Can you work these out from the model? Positions are in its coordinate system, mm. A direction names the side the tool comes from. Give positions to 0.01 mm unless a question says otherwise; leave off trailing zeros. Use a Markdown table: item, result. Add a question column.
```python
from build123d import *

# Parameters (mm, degrees)
F0_W      = 2.5
F0_H      = 4.3
F1_DEPTH  = 0.01
F4_W      = 3
F4_H      = 2.4
F5_DEPTH  = 2
F0_W_2    = 0.25
F0_H_2    = 26.2
F6_DEPTH  = 0.01
F7_DEPTH  = 0.01
F7_FACE_W = 0.25
F7_FACE_H = 28.7
F6_FACE_W = 0.25
F6_FACE_H = 26.2
F10_R     = 0.2
F11_W     = 38
F11_H     = 33
F12_DEPTH = 12.5


with BuildPart() as f1:
    # F0 (on Front) → F1 (new body)
    with BuildSketch(Plane.XZ):
        with Locations((1.25, 2.15)):
            Rectangle(F0_W, F0_H)
        Polygon((2.5, 0), (0, 0), (0, -1), (1.02, -1), (1.27, -1), (2.9, -1), (2.9, 0), align=None)
    extrude(amount=F1_DEPTH)

    # F1_face (on face) → F2 (revolve)
    with BuildSketch(Plane(origin=(1.2924908425, -0.01, 1.586996337), x_dir=(1, 0, 0), z_dir=(0, -1, 0))):
        Polygon((-1.2924908425, 2.713003663), (-1.2924908425, -2.586996337), (1.6075091575, -2.586996337), (1.6075091575, -1.586996337), (1.2075091575, -1.586996337), (1.2075091575, 2.713003663), align=None)
    revolve(axis=Axis((0, 0, 1.65), (0, 0, 1)))

    # F4 (on offset) → F5 (cut)
    with BuildSketch(Plane.YZ.offset(2.5)):
        Rectangle(F4_W, F4_H)
    extrude(amount=F5_DEPTH, mode=Mode.SUBTRACT)

    # F0 (on Front) → F6 (join)
    with BuildSketch(Plane.XZ):
        with Locations((1.145, -14.1)):
            Rectangle(F0_W_2, F0_H_2)
    extrude(amount=F6_DEPTH)

    # F0 (on Front) → F7 (join)
    with BuildSketch(Plane.XZ):
        Polygon((-1.02, -29.7), (-1.02, -27.2), (-1.02, -1), (-1.27, -1), (-1.27, -29.7), align=None)
    extrude(amount=F7_DEPTH)

    # F7_face (on face) → F8 (revolve)
    with BuildSketch(Plane(origin=(-1.145, -0.01, -15.35), x_dir=(1, 0, 0), z_dir=(0, -1, 0))):
        Rectangle(F7_FACE_W, F7_FACE_H)
    revolve(axis=Axis((-1.27, 0, -15.35), (0, 0, 1)))

    # F6_face (on face) → F9 (revolve)
    with BuildSketch(Plane(origin=(1.145, -0.01, -14.1), x_dir=(1, 0, 0), z_dir=(0, -1, 0))):
        Rectangle(F6_FACE_W, F6_FACE_H)
    revolve(axis=Axis((1.27, 0, -14.1), (0, 0, -1)))

    # F10
    f10_edges = [f1.edges().sort_by_distance(p)[0] for p in [
        (-2.5, 0.01, 4.3),
    ]]
    fillet(f10_edges, radius=F10_R)

    # F11 (on Front) → F12 (cut, symmetric)
    with BuildSketch(Plane.XZ):
        with Locations((1.6585592992, -18.5)):
            Rectangle(F11_W, F11_H)
    extrude(amount=F12_DEPTH, both=True, mode=Mode.SUBTRACT)


solid = f1.part
```
Q1. If I drill on probe 1 along Z at (x, y) = (-1.55, -2.25); probe 2 along Z at (x, y) = (0.4, -2.1); probe 3 along Y at (x, z) = (0.75, 1), over which ranges is the centre line in solid material (lowest first)? Write a range as [from, to].
Q2. On a 3-axis mill with a long thin cutter (end or side, diameter ignored), from which of +Z, -Z, +X, -X, +Y, -Y can I reach the whole of each face in a straight line? I mean faces 1 (the cylindrical face through (-2.9, 0.1, -0.5)), 2 (the cylindrical face through (2.306, -0.967, 2.079)). Say none if no direction works.
Q3. Suppose I cut it at A-A (z = -1.5). Give the number of separate pieces and of enclosed holes in the cut face, and give its area (3 significant figures).
Q4. I'm going to push a flat-ended pin straight in: P1, Ø1, axis at y = 1, z = 3, coming from the +X side. Where does the tip first touch, or does it pass through?
Derived:
| question | item | result |
|---|---|---|
| 1 | probe 1 | [-1, 0] |
| 1 | probe 2 | [-1, 4.3] |
| 1 | probe 3 | [-2.38, 2.38] |
| 2 | face 1 | +Z, -Z |
| 2 | face 2 | +Z |
| 3 | separate pieces | 2 |
| 3 | enclosed holes | 2 |
| 3 | area | 0.393 mm² |
| 4 | P1 | x = 2.45 |
